Read the model definition and answer for the solid it produces. Units are mm, in the model's axes. A direction names the side the tool comes from. Coordinates: 2 decimals unless noted, no trailing zeros. Order: outer loops, then holes, each group sorted by start corner. A loop starts at its lowest first (then second) coordinate and runs counter-clockwise, first axis right, second up. Notation, with made-up numbers: (3, 23) - (24, 23) arc R21 ccw to (24, 49) - close; hole circle Ø9 at (77.25, -25.5). An arc over 180 degrees is marked (long way). Use one line per item in the form item = value. Start each with the question number.
from build123d import *

# Parameters (mm, degrees)
BOX763_W           = 148
BOX763_H           = 74
BOX763_DEPTH       = 55
CYLINDER1803_R     = 2.5
CYLINDER1803_DEPTH = 20
CYLINDER1804_R     = 2.5
CYLINDER1804_DEPTH = 20
CYLINDER1802_R     = 74
CYLINDER1802_DEPTH = 32
BOX762_W           = 68
BOX762_H           = 56
BOX762_DEPTH       = 6
CHAMFER063_SIZE    = 20


with BuildPart() as krychle763:
    # Box763 → Box763 (new body)
    with BuildSketch(Plane(origin=(-74, 0, 29), x_dir=(1, 0, 0), z_dir=(0, 0, 1))):
        with Locations((74, 37)):
            Rectangle(BOX763_W, BOX763_H)
    extrude(amount=BOX763_DEPTH)


with BuildPart() as obj1:
    # Cylinder1803 → Cylinder1803 (new body)
    with BuildSketch(Plane(origin=(-90, -10, 66), x_dir=(1, 0, 0), z_dir=(0, 0, 1))):
        Circle(CYLINDER1803_R)
    extrude(amount=CYLINDER1803_DEPTH)


with BuildPart() as compound921:
    # Cylinder1804 → Cylinder1804 (new body)
    with BuildSketch(Plane(origin=(-110, -10, 66), x_dir=(1, 0, 0), z_dir=(0, 0, 1))):
        Circle(CYLINDER1804_R)
    extrude(amount=CYLINDER1804_DEPTH)

    # Compound921: union obj1
    add(obj1.part)


with BuildPart() as compound921_1:
    # Compound921 placement: moved
    add(compound921.part.moved(Location((-8, 0, 0))))


with BuildPart() as obj2:
    # Cylinder1802 → Cylinder1802 (new body)
    with BuildSketch(Plane.XY.offset(66)):
        Circle(CYLINDER1802_R)
    extrude(amount=CYLINDER1802_DEPTH)


with BuildPart() as cut566:
    # Box762 → Box762 (new body)
    with BuildSketch(Plane(origin=(-130, -24, 76), x_dir=(1, 0, 0), z_dir=(0, 0, 1))):
        with Locations((34, 28)):
            Rectangle(BOX762_W, BOX762_H)
    extrude(amount=BOX762_DEPTH)

    # Cut561: cut obj2
    add(obj2.part, mode=Mode.SUBTRACT)

    # Cut562: cut Compound921
    add(compound921_1.part, mode=Mode.SUBTRACT)


with BuildPart() as cut566_1:
    # Cut562 placement: moved
    add(cut566.part.moved(Location((0, 0, 2))))

    # Chamfer063
    chamfer063_edges = [cut566_1.edges().sort_by_distance(p)[0] for p in [
        (-130, 32, 81),
    ]]
    chamfer(chamfer063_edges, length=CHAMFER063_SIZE)

    # Cut566: cut Krychle763
    add(krychle763.part, mode=Mode.SUBTRACT)


solid = cut566_1.part
Q1. Given P1, Ø1, axis at y = -4.5, z = 81.5, coming from the +X side; P2, Ø1, axis at x = -114, z = 82.5, coming from the +Y side, each flat-ended and moving along its own axis, determine where each tip first touches the part or whether it passes through.
Q2. A cutting plane is placed at A-A (x = -98). Give the vertices of the cut face in (y, z), then the cut area to 3 significant figures.
Q3. Consider probe 1 along Y at (x, z) = (-98, 79.35); probe 2 along X at (y, z) = (-10, 81.75); probe 3 along X at (y, z) = (9, 81.1). Determine where each line is inside the solid, lowest interval first.
Q4. A cutting plane is placed at C-C (z = 81.4). Give the vertices of the cut face in (x, y), then the cut area to 3 significant figures.
Q5. Which of the six approach directions +Z, -Z, +X, -X, +Y, -Y give full straight-line access (tool end or side, diameter ignored) to faces 1 (the flat face through (-120, 22, 81)), 2 (the flat face through (-74, 16, 81))?
Q6. For a pull along X with two mould halves and no side action, classify faces 3 (the flat face through (-100, 4, 84)), 4 (the cylindrical face through (-100, -11.5, 81)), 5 (the flat face through (-130, -6, 81)) as +X half, -X half, draft (parallel to the pull), parting line (faces both ways), or undercut.
Q7. A cutting plane is placed at B-B (y = -10). Give the vertices of the cut face in (x, z), then the cut area to 3 significant figures.
Q8. A cutting plane is placed at D-D (x = -118). Give the vertices of the cut face in (y, z).
Result sheet:
q1.P1 = -73.83
q1.P2 = 28.5
q2.outline = (-24, 78) - (-12.5, 78) - (-12.5, 84) - (-24, 84) - close; (-7.5, 78) - (32, 78) - (32, 84) - (-7.5, 84) - close
q2.area = 306 mm^2
q3.probe_1 = -24 to -12.5, -7.5 to 32
q3.probe_2 = -130 to -120.5, -115.5 to -100.5, -95.5 to -73.32
q3.probe_3 = -130 to -74
q4.outline = (-130, -24) - (-70, -24) arc R74 cw to (-74, 0) - (-74, 32) - (-110, 32) - (-130, 12) - close; hole circle Ø5 at (-118, -10); hole circle Ø5 at (-98, -10)
q4.area = 2,930 mm^2
q5.face_1 = +Z, -Z, -X, +Y
q5.face_2 = +Z, -Z, +X, +Y
q6.face_3 = draft
q6.face_4 = undercut
q6.face_5 = -X half
q7.outline = (-130, 78) - (-120.5, 78) - (-120.5, 84) - (-130, 84) - close; (-115.5, 78) - (-100.5, 78) - (-100.5, 84) - (-115.5, 84) - close; (-95.5, 78) - (-73.32, 78) - (-73.32, 84) - (-95.5, 84) - close
q7.area = 280 mm^2
q8.outline = (-24, 78) - (-12.5, 78) - (-12.5, 84) - (-24, 84) - close; (-7.5, 78) - (24, 78) - (24, 84) - (-7.5, 84) - close
